```python
from build123d import *

# Parameters (mm, degrees)
F1_DEPTH  = 50.8
F2_R      = 5.08
F1_FACE_W = 116.832122
F1_FACE_H = 45.72
F3_DEPTH  = 75.692
F5_D      = 5


with BuildPart() as f1:
    # F0 (on Top) → F1 (new body)
    with BuildSketch(Plane.XY):
        Polygon((-2.999169, 76.140955), (0, 0), (127, 0), (124.000831, 76.140955), align=None)
    extrude(amount=F1_DEPTH)

    # F2
    f2_edges = [f1.edges().sort_by_distance(p)[0] for p in [
        (63.5, 0, 50.8),
        (125.500415, 38.070477, 50.8),
        (127, 0, 25.4),
        (0, 0, 25.4),
        (-1.499585, 38.070477, 50.8),
    ]]
    fillet(f2_edges, radius=F2_R)

    # F1_face (on face) → F3 (cut)
    with BuildSketch(Plane(origin=(63.2999, 0, 22.86), x_dir=(1, 0, 0), z_dir=(0, -1, 0))):
        Rectangle(F1_FACE_W, F1_FACE_H)
    extrude(amount=-F3_DEPTH, mode=Mode.SUBTRACT)

    # F5 (through all)
    with Locations(Plane.XY.offset(50.8)):
        with Locations((6.445575, 71.227975)):
            Hole(F5_D / 2)


solid = f1.part
```
The model under review builds one solid part; all positions refer to its coordinate system, in mm. A direction names the side the tool comes from. Give positions to 0.01 mm unless a question says otherwise; leave off trailing zeros. Write each loop counter-clockwise with the first axis right and the second up, starting at its lowest first coordinate (ties: lowest second). Pieces come first, ordered by that corner, then holes.
(1) For P1, Ø2, axis at x = 52.5, z = 17, coming from the -Y side; P2, Ø8, axis at y = 23.5, z = 5.5, coming from the -X side; P3, Ø12, axis at y = 21, z = 43.5, coming from the +X side, all flat-tipped, find the tip position at first contact; note any pin that passes through.
(2) Consider section A-A, the plane z = 29. Give the boundary of the cut face in (x, y), and give its area (3 significant figures).
(3) Consider section B-B, the plane x = 53. Give the boundary of the cut face in (y, z).
(4) To check wall thickness, follow L1, parallel to Y at x = 121, z = 19; L2, parallel to Z at x = 100, y = 30.5; L3, parallel to X at y = 15, z = 30.5. State the ranges of each line that lie inside material, in increasing order.
(5) The part is to be moulded in two halves that separate along X. For faces 1 (the flat face through (62, 75.692, 23)), 2 (the cylindrical face through (1.32, 1.46, 23.18)), 3 (the flat face through (4.884, 74, 23)), 4 (the flat face through (4, 41, 0)), say which applies: released by +X, released by -X, zero draft, split by the parting line, or undercut.
(6) Tool access review of faces 5 (the flat face through (61, 41, 50.8)), 6 (the flat face through (62, 37, 45.72)): name each direction out of +Z, -Z, +X, -X, +Y, -Y from which nothing blocks a thin tool from reaching the whole face with its end or side.
Returned:
1. P1: stops at y = 75.69
1. P2: stops at x = -1.08
1. P3: stops at x = 126.41
2. outline: (-3, 76.14) - (-0.19, 4.88) arc R5.08 ccw to (4.88, 0) - (4.88, 69.28) arc R2.5 cw to (4.88, 73.18) - (4.88, 75.69) - (121.72, 75.69) - (121.72, 0) arc R5.08 ccw to (126.79, 5.28) - (124, 76.14) - close
2. area: 813 mm2
3. outline: (0, 45.72) - (75.69, 45.72) - (75.69, 0) - (76.14, 0) - (76.14, 50.8) - (5.08, 50.8) arc R5.08 ccw to start
4. L1: y = 75.69 to 76.14
4. L2: z = 45.72 to 50.8
4. L3: x = -0.59 to 4.88, 121.72 to 126.41
5. face 1: undercut
5. face 2: released by -X
5. face 3: undercut
5. face 4: zero draft
6. face 5: +Z, +X, -X, +Y, -Y
6. face 6: -Z, -Y
